```python
from build123d import *

# Parameters (mm, degrees)
SKETCH1_W               = 76
SKETCH1_H               = 223.60679775
BOSS_EXTRUDE1_DEPTH     = 1.61
SKETCH2_W               = 3.22
SKETCH2_H               = 12
CUT_EXTRUDE1_DEPTH      = 3.22
LPATTERN1_COUNT         = 10
LPATTERN1_PITCH         = 24
MIRROR1_COPY_1_SKETCH_W = 3.22
MIRROR1_COPY_1_SKETCH_H = 12
MIRROR1_COPY_1_DEPTH    = 3.22
MIRROR1_COPY_2_SKETCH_W = 3.22
MIRROR1_COPY_2_SKETCH_H = 12
MIRROR1_COPY_2_DEPTH    = 3.22
MIRROR1_COPY_3_SKETCH_W = 3.22
MIRROR1_COPY_3_SKETCH_H = 12
MIRROR1_COPY_3_DEPTH    = 3.22
MIRROR1_COPY_4_SKETCH_W = 3.22
MIRROR1_COPY_4_SKETCH_H = 12
MIRROR1_COPY_4_DEPTH    = 3.22
MIRROR1_COPY_5_SKETCH_W = 3.22
MIRROR1_COPY_5_SKETCH_H = 12
MIRROR1_COPY_5_DEPTH    = 3.22
MIRROR1_COPY_6_SKETCH_W = 3.22
MIRROR1_COPY_6_SKETCH_H = 12
MIRROR1_COPY_6_DEPTH    = 3.22
MIRROR1_COPY_7_SKETCH_W = 3.22
MIRROR1_COPY_7_SKETCH_H = 12
MIRROR1_COPY_7_DEPTH    = 3.22
MIRROR1_COPY_8_SKETCH_W = 3.22
MIRROR1_COPY_8_SKETCH_H = 12
MIRROR1_COPY_8_DEPTH    = 3.22
MIRROR1_COPY_9_SKETCH_W = 3.22
MIRROR1_COPY_9_SKETCH_H = 12
MIRROR1_COPY_9_DEPTH    = 3.22
SKETCH4_R               = 5.5
CUT_EXTRUDE2_DEPTH      = 10
CUT_EXTRUDE5_REACH      = 5.22
SKETCH7_W               = 3.22
SKETCH7_H               = 20
CUT_EXTRUDE7_DEPTH      = 3.22
LPATTERN2_COUNT         = 6
LPATTERN2_PITCH         = 24


with BuildPart() as part:
    # Sketch1 → Boss-Extrude1 (new body, symmetric)
    with BuildSketch(Plane(origin=(0, 0, 0), x_dir=(1, 0, 0), z_dir=(0, 1, 0))):
        Rectangle(SKETCH1_W, SKETCH1_H)
    extrude(amount=BOSS_EXTRUDE1_DEPTH, both=True)

    # Sketch2 → Cut-Extrude1 (cut)
    with BuildSketch(Plane(origin=(0, 1.61, 0), x_dir=(1, 0, 0), z_dir=(0, 1, 0))):
        with Locations((36.39, 105.803398875)):
            Rectangle(SKETCH2_W, SKETCH2_H)
    cut_extrude1 = extrude(amount=-CUT_EXTRUDE1_DEPTH, mode=Mode.SUBTRACT)

    # LPattern1: Cut-Extrude1 ×10
    with Locations(*[(0, 0, i * LPATTERN1_PITCH) for i in range(1, LPATTERN1_COUNT)]):
        add(cut_extrude1, mode=Mode.SUBTRACT)

    # Mirror1: Cut-Extrude1 across plane
    add(cut_extrude1.mirror(Plane(origin=(0, 0, 0), x_dir=(0, 0, 1), z_dir=(1, 0, 0))), mode=Mode.SUBTRACT)

    # Mirror1 copy 1 sketch → Mirror1 copy 1 (cut)
    with BuildSketch(Plane(origin=(0, 1.61, 24), x_dir=(-1, 0, 0), z_dir=(0, 1, 0))):
        with Locations((36.39, -105.803398875)):
            Rectangle(MIRROR1_COPY_1_SKETCH_W, MIRROR1_COPY_1_SKETCH_H)
    extrude(amount=-MIRROR1_COPY_1_DEPTH, mode=Mode.SUBTRACT)

    # Mirror1 copy 2 sketch → Mirror1 copy 2 (cut)
    with BuildSketch(Plane(origin=(0, 1.61, 48), x_dir=(-1, 0, 0), z_dir=(0, 1, 0))):
        with Locations((36.39, -105.803398875)):
            Rectangle(MIRROR1_COPY_2_SKETCH_W, MIRROR1_COPY_2_SKETCH_H)
    extrude(amount=-MIRROR1_COPY_2_DEPTH, mode=Mode.SUBTRACT)

    # Mirror1 copy 3 sketch → Mirror1 copy 3 (cut)
    with BuildSketch(Plane(origin=(0, 1.61, 72), x_dir=(-1, 0, 0), z_dir=(0, 1, 0))):
        with Locations((36.39, -105.803398875)):
            Rectangle(MIRROR1_COPY_3_SKETCH_W, MIRROR1_COPY_3_SKETCH_H)
    extrude(amount=-MIRROR1_COPY_3_DEPTH, mode=Mode.SUBTRACT)

    # Mirror1 copy 4 sketch → Mirror1 copy 4 (cut)
    with BuildSketch(Plane(origin=(0, 1.61, 96), x_dir=(-1, 0, 0), z_dir=(0, 1, 0))):
        with Locations((36.39, -105.803398875)):
            Rectangle(MIRROR1_COPY_4_SKETCH_W, MIRROR1_COPY_4_SKETCH_H)
    extrude(amount=-MIRROR1_COPY_4_DEPTH, mode=Mode.SUBTRACT)

    # Mirror1 copy 5 sketch → Mirror1 copy 5 (cut)
    with BuildSketch(Plane(origin=(0, 1.61, 120), x_dir=(-1, 0, 0), z_dir=(0, 1, 0))):
        with Locations((36.39, -105.803398875)):
            Rectangle(MIRROR1_COPY_5_SKETCH_W, MIRROR1_COPY_5_SKETCH_H)
    extrude(amount=-MIRROR1_COPY_5_DEPTH, mode=Mode.SUBTRACT)

    # Mirror1 copy 6 sketch → Mirror1 copy 6 (cut)
    with BuildSketch(Plane(origin=(0, 1.61, 144), x_dir=(-1, 0, 0), z_dir=(0, 1, 0))):
        with Locations((36.39, -105.803398875)):
            Rectangle(MIRROR1_COPY_6_SKETCH_W, MIRROR1_COPY_6_SKETCH_H)
    extrude(amount=-MIRROR1_COPY_6_DEPTH, mode=Mode.SUBTRACT)

    # Mirror1 copy 7 sketch → Mirror1 copy 7 (cut)
    with BuildSketch(Plane(origin=(0, 1.61, 168), x_dir=(-1, 0, 0), z_dir=(0, 1, 0))):
        with Locations((36.39, -105.803398875)):
            Rectangle(MIRROR1_COPY_7_SKETCH_W, MIRROR1_COPY_7_SKETCH_H)
    extrude(amount=-MIRROR1_COPY_7_DEPTH, mode=Mode.SUBTRACT)

    # Mirror1 copy 8 sketch → Mirror1 copy 8 (cut)
    with BuildSketch(Plane(origin=(0, 1.61, 192), x_dir=(-1, 0, 0), z_dir=(0, 1, 0))):
        with Locations((36.39, -105.803398875)):
            Rectangle(MIRROR1_COPY_8_SKETCH_W, MIRROR1_COPY_8_SKETCH_H)
    extrude(amount=-MIRROR1_COPY_8_DEPTH, mode=Mode.SUBTRACT)

    # Mirror1 copy 9 sketch → Mirror1 copy 9 (cut)
    with BuildSketch(Plane(origin=(0, 1.61, 216), x_dir=(-1, 0, 0), z_dir=(0, 1, 0))):
        with Locations((36.39, -105.803398875)):
            Rectangle(MIRROR1_COPY_9_SKETCH_W, MIRROR1_COPY_9_SKETCH_H)
    extrude(amount=-MIRROR1_COPY_9_DEPTH, mode=Mode.SUBTRACT)

    # Sketch4 → Cut-Extrude2 (cut)
    with BuildSketch(Plane.XZ.offset(1.61)):
        with Locations((-20, -98.803398875)):
            Circle(SKETCH4_R)
        with Locations((20, -98.803398875)):
            Circle(SKETCH4_R)
    extrude(amount=-CUT_EXTRUDE2_DEPTH, mode=Mode.SUBTRACT)

    # Sketch7 → Cut-Extrude5 (cut, up to next)
    with BuildSketch(Plane.XZ.offset(1.61), mode=Mode.PRIVATE) as cut_extrude5_sk1:
        with Locations((-11.27, 95.803398875)):
            Rectangle(SKETCH7_W, SKETCH7_H)
    cut_extrude5_tool1 = extrude(cut_extrude5_sk1.sketch, amount=-CUT_EXTRUDE5_REACH, mode=Mode.PRIVATE) & part.part
    add(cut_extrude5_tool1.solids().sort_by_distance((-11.27, -1.61, 95.803399))[0], mode=Mode.SUBTRACT)
    # Sketch7 → Cut-Extrude5 (cut, up to next)
    with BuildSketch(Plane.XZ.offset(1.61), mode=Mode.PRIVATE) as cut_extrude5_sk2:
        with Locations((-4.83, 95.803398875)):
            Rectangle(SKETCH7_W, SKETCH7_H)
    cut_extrude5_tool2 = extrude(cut_extrude5_sk2.sketch, amount=-CUT_EXTRUDE5_REACH, mode=Mode.PRIVATE) & part.part
    add(cut_extrude5_tool2.solids().sort_by_distance((-4.83, -1.61, 95.803399))[0], mode=Mode.SUBTRACT)
    # Sketch7 → Cut-Extrude5 (cut, up to next)
    with BuildSketch(Plane.XZ.offset(1.61), mode=Mode.PRIVATE) as cut_extrude5_sk3:
        with Locations((4.83, 95.803398875)):
            Rectangle(SKETCH7_W, SKETCH7_H)
    cut_extrude5_tool3 = extrude(cut_extrude5_sk3.sketch, amount=-CUT_EXTRUDE5_REACH, mode=Mode.PRIVATE) & part.part
    add(cut_extrude5_tool3.solids().sort_by_distance((4.83, -1.61, 95.803399))[0], mode=Mode.SUBTRACT)
    # Sketch7 → Cut-Extrude5 (cut, up to next)
    with BuildSketch(Plane.XZ.offset(1.61), mode=Mode.PRIVATE) as cut_extrude5_sk4:
        with Locations((11.27, 95.803398875)):
            Rectangle(SKETCH7_W, SKETCH7_H)
    cut_extrude5_tool4 = extrude(cut_extrude5_sk4.sketch, amount=-CUT_EXTRUDE5_REACH, mode=Mode.PRIVATE) & part.part
    add(cut_extrude5_tool4.solids().sort_by_distance((11.27, -1.61, 95.803399))[0], mode=Mode.SUBTRACT)

    # Sketch8 → Cut-Extrude7 (cut)
    with BuildSketch(Plane(origin=(0, 1.61, 0), x_dir=(1, 0, 0), z_dir=(0, 1, 0))):
        Polygon((-5.2, 60), (-15.303629711, 77.5), (-25.407259422, 60), align=None)
        Polygon((-10.103629711, 77.5), (10.103629711, 77.5), (0, 60), align=None)
        Polygon((15.303629711, 77.5), (25.407259422, 60), (5.2, 60), align=None)
    cut_extrude7 = extrude(amount=-CUT_EXTRUDE7_DEPTH, mode=Mode.SUBTRACT)

    # LPattern2: Cut-Extrude7 ×6
    with Locations(*[(0, 0, i * LPATTERN2_PITCH) for i in range(1, LPATTERN2_COUNT)]):
        add(cut_extrude7, mode=Mode.SUBTRACT)


solid = part.part
```
Here's how the part is built. I have some questions about the finished solid (model axes, mm). Coordinates: 2 decimals unless noted, no trailing zeros. Order: outer loops, then holes, each group sorted by start corner. A loop starts at its lowest first (then second) coordinate and runs counter-clockwise, first axis right, second up.
1) I need wall thicknesses on line 1 (X direction, y = -0.9, z = 92); line 2 (X direction, y = -1.05, z = -45.5); line 3 (X direction, y = 0.5, z = -101). Which ranges of each line are inside material? Lowest first, please.
2) Imagine slicing it at A-A on z = 28.5. List the corners of the cut face in (x, y) for me.
3) Imagine slicing it at B-B on x = -20. State how many separate pieces and enclosed holes the cut face has, and give its area (3 significant figures).
4) Will these pins go through, and if not, where does the flat tip stop? pin 1 (1 mm diameter, centred on y = -0.5, z = -10, fed in from -X); pin 2 (1.6 mm diameter, centred on x = 36.5, y = -0.5, fed in from +Z); pin 3 (1.6 mm diameter, centred on x = -36.5, y = -0.5, fed in from -Z).
Response values:
1. line 1: x = -34.78 to -12.88, -9.66 to -6.44, -3.22 to 3.22, 6.44 to 9.66, 12.88 to 34.78
1. line 2: x = -38 to -19.92, -10.68 to -5.48, 5.48 to 10.68, 19.92 to 38
1. line 3: x = -34.78 to -25.04, -14.96 to 14.96, 25.04 to 34.78
2. outline: (-38, -1.61) - (-21.08, -1.61) - (-21.08, 1.61) - (-38, 1.61) - close; (-9.53, -1.61) - (-4.33, -1.61) - (-4.33, 1.61) - (-9.53, 1.61) - close; (4.33, -1.61) - (9.53, -1.61) - (9.53, 1.61) - (4.33, 1.61) - close; (21.08, -1.61) - (38, -1.61) - (38, 1.61) - (21.08, 1.61) - close
3. separate pieces: 8
3. enclosed holes: 0
3. area: 504 mm2
4. pin 1: stops at x = -34.78
4. pin 2: stops at z = 104.2
4. pin 3: stops at z = -99.8
